from build123d import *

# Parameters (mm, degrees)
BOSS_EXTRUDE1_DEPTH = 20
SKETCH5_R           = 5.25
CUT_EXTRUDE4_DEPTH  = 20
SKETCH6_W           = 13
SKETCH6_H           = 13
CUT_EXTRUDE5_DEPTH  = 15.5
SKETCH7_W           = 13
SKETCH7_H           = 13
CUT_EXTRUDE6_DEPTH  = 15.5
SKETCH8_W           = 300
SKETCH8_H           = 102
BOSS_EXTRUDE2_DEPTH = 20
CUT_EXTRUDE7_START  = -150
SKETCH9_W           = 47.842391085
SKETCH9_H           = 20
CUT_EXTRUDE7_DEPTH  = 150
CUT_EXTRUDE9_DEPTH  = 40
CUT_EXTRUDE10_DEPTH = 60
SKETCH17_W          = 60
SKETCH17_H          = 5
CUT_EXTRUDE12_DEPTH = 38
CUT_EXTRUDE13_DEPTH = 60
SKETCH10_W          = 252.157608915
SKETCH10_H          = 50
CUT_EXTRUDE8_DEPTH  = 310
BOSS_EXTRUDE3_DEPTH = 50
SKETCH21_W          = 252.157608915
SKETCH21_H          = 10
CUT_EXTRUDE14_DEPTH = 54
SKETCH23_W          = 60
SKETCH23_H          = 5
BOSS_EXTRUDE5_DEPTH = 20
CUT_EXTRUDE15_DEPTH = 20
SKETCH22_W          = 60
SKETCH22_H          = 5
BOSS_EXTRUDE4_DEPTH = 20


with BuildPart() as part:
    # Sketch1 → Boss-Extrude1 (new body)
    with BuildSketch(Plane.XY):
        Polygon((-107.821386225, 92.09039548), (-7.821386225, 92.09039548), (117.178613775, 92.09039548), (117.178613775, 44.09039548), (-7.821386225, 44.09039548), (-107.821386225, 44.09039548), (-182.821386225, 44.09039548), (-182.821386225, 92.09039548), align=None)
    extrude(amount=BOSS_EXTRUDE1_DEPTH)

    # Sketch5 → Cut-Extrude4 (cut)
    with BuildSketch(Plane(origin=(0, 92.09039548, 0), x_dir=(1, 0, 0), z_dir=(0, 1, 0))):
        with Locations(Location((-66.321386225, -10, 0), (0, 0, 180))):
            Circle(SKETCH5_R)
        with Locations(Location((-47.321386225, -10, 0), (0, 0, 180))):
            Circle(SKETCH5_R)
    extrude(amount=-CUT_EXTRUDE4_DEPTH, mode=Mode.SUBTRACT)

    # Sketch6 → Cut-Extrude5 (cut)
    with BuildSketch(Plane(origin=(0, 92.09039548, 0), x_dir=(1, 0, 0), z_dir=(0, 1, 0))):
        with Locations((-99.441386225, -10.25)):
            Rectangle(SKETCH6_W, SKETCH6_H)
    extrude(amount=-CUT_EXTRUDE5_DEPTH, mode=Mode.SUBTRACT)

    # Sketch7 → Cut-Extrude6 (cut)
    with BuildSketch(Plane(origin=(0, 92.09039548, 0), x_dir=(1, 0, 0), z_dir=(0, 1, 0))):
        with Locations((-14.16377731, -10.25)):
            Rectangle(SKETCH7_W, SKETCH7_H)
    extrude(amount=-CUT_EXTRUDE6_DEPTH, mode=Mode.SUBTRACT)

    # Sketch8 → Boss-Extrude2 (add)
    with BuildSketch(Plane.XY.offset(20)):
        with Locations((-32.821386225, -6.90960452)):
            Rectangle(SKETCH8_W, SKETCH8_H)
    extrude(amount=-BOSS_EXTRUDE2_DEPTH)

    # Sketch9 → Cut-Extrude7 (cut)
    with BuildSketch(Plane(origin=(0, 92.09039548, 0), x_dir=(1, 0, 0), z_dir=(0, 1, 0)).offset(CUT_EXTRUDE7_START)):
        with Locations((93.257418233, -10)):
            Rectangle(SKETCH9_W, SKETCH9_H)
    extrude(amount=CUT_EXTRUDE7_DEPTH, mode=Mode.SUBTRACT)

    # Sketch11 → Cut-Extrude9 (cut)
    with BuildSketch(Plane.XY.offset(20)):
        Polygon((-26.742581768, 62.09039548), (-26.742581768, 12.09039548), (-86.742581768, 12.09039548), (-86.742581768, 62.09039548), (-86.742581768, 64.09039548), (-26.742581768, 64.09039548), align=None)
    extrude(amount=-CUT_EXTRUDE9_DEPTH, mode=Mode.SUBTRACT)

    # Sketch14 → Cut-Extrude10 (cut)
    with BuildSketch(Plane(origin=(-86.742581768, 0, 0), x_dir=(0, 0, -1), z_dir=(1, 0, 0))):
        Polygon((0, 64.09039548), (-20, 67.09039548), (-20, 64.09039548), align=None)
    extrude(amount=CUT_EXTRUDE10_DEPTH, mode=Mode.SUBTRACT)

    # Sketch17 → Cut-Extrude12 (cut)
    with BuildSketch(Plane(origin=(0, 0, 0), x_dir=(-1, 0, 0), z_dir=(0, 0, -1))):
        with Locations((56.742581768, 89.59039548)):
            Rectangle(SKETCH17_W, SKETCH17_H)
    extrude(amount=-CUT_EXTRUDE12_DEPTH, mode=Mode.SUBTRACT)

    # Sketch19 → Cut-Extrude13 (cut)
    with BuildSketch(Plane.ZY.offset(26.742581768)):
        Polygon((0, 12.09039548), (2, 12.09039548), (8, -57.90960452), (0, -57.90960452), align=None)
    extrude(amount=CUT_EXTRUDE13_DEPTH, mode=Mode.SUBTRACT)

    # Sketch10 → Cut-Extrude8 (cut)
    with BuildSketch(Plane(origin=(0, 0, 0), x_dir=(-1, 0, 0), z_dir=(0, 0, -1))):
        with Locations((56.742581767, -32.90960452)):
            Rectangle(SKETCH10_W, SKETCH10_H)
    extrude(amount=-CUT_EXTRUDE8_DEPTH, mode=Mode.SUBTRACT)

    # Sketch20 → Boss-Extrude3 (add)
    with BuildSketch(Plane.XZ.offset(7.90960452)):
        Polygon((69.33622269, 20), (-182.821386225, 20), (-182.821386225, 0), (-86.742581768, 0), (-86.742581768, 3.714285714), (-26.742581768, 3.714285714), (-26.742581768, 0), (69.33622269, 0), align=None)
    extrude(amount=BOSS_EXTRUDE3_DEPTH)

    # Sketch21 → Cut-Extrude14 (cut)
    with BuildSketch(Plane.XY.offset(20)):
        with Locations((-56.742581767, -52.90960452)):
            Rectangle(SKETCH21_W, SKETCH21_H)
    extrude(amount=-CUT_EXTRUDE14_DEPTH, mode=Mode.SUBTRACT)

    # Sketch23 → Boss-Extrude5 (add)
    with BuildSketch(Plane.XY.offset(20)):
        with Locations((-56.742581768, 89.59039548)):
            Rectangle(SKETCH23_W, SKETCH23_H)
    extrude(amount=-BOSS_EXTRUDE5_DEPTH)

    # Sketch24 → Cut-Extrude15 (cut)
    with BuildSketch(Plane.XY.offset(20)):
        Polygon((-86.742581768, 67.09039548), (-86.742581768, 72.09039548), (-26.742581768, 72.09039548), (-26.742581768, 67.09039548), (-26.742581768, 61.01073747), (-86.742581768, 61.01073747), align=None)
    extrude(amount=-CUT_EXTRUDE15_DEPTH, mode=Mode.SUBTRACT)

    # Sketch22 → Boss-Extrude4 (add)
    with BuildSketch(Plane.XY.offset(20)):
        with Locations((-56.742581768, 89.59039548)):
            Rectangle(SKETCH22_W, SKETCH22_H)
    extrude(amount=-BOSS_EXTRUDE4_DEPTH)


solid = part.part
For this review, take the finished solid that the model builds, in its own axes (mm). A direction names the side the tool comes from. Round coordinates to 2 decimals unless told otherwise and drop trailing zeros. Order: outer loops, then holes, each group sorted by start corner. A loop starts at its lowest first (then second) coordinate and runs counter-clockwise, first axis right, second up. Notation, with made-up numbers: M 83,63.25 L 141,63.25 A27 cw 141,99.25 Z; hole C 36,-21.5 d5. An arc over 180 degrees is marked long. Write each question's results on one line, items separated by ' | '. Start each with the question number.
1. To check wall thickness, follow L1, parallel to X at y = 68, z = 6.5; L2, parallel to Y at x = -79.5, z = 4.5; L3, parallel to Y at x = -71, z = 12. State the ranges of each line that lie inside material, in increasing order. Write a range as [from, to].
2. Add section C-C (y = 66). State the section outline as (x, z) points, then the cut area to 3 significant figures.
3. Tool access review of faces 4 (the face through (-100, 84, 3.75)), 5 (the face through (-57, 72.09, 10)), 6 (the face through (-71.33, 79.7, 11.58)): name each direction out of +Z, -Z, +X, -X, +Y, -Y from which nothing blocks a thin tool from reaching the whole face with its end or side.
4. Draft analysis for pull direction Z (two halves, no side actions). For faces 1 (the face through (-56.323, 2.23, 2.845)), 2 (the face through (-26.743, 26, 10)), 3 (the face through (-66, 87.09, 10)), state which applies: pulls with the +Z half, pulls with the -Z half, needs draft (parallel to the pull), parting line crosses it, or undercut.
5. Add section A-A (x = -79.5). State the section outline as (y, z) points.
6. Add section D-D (y = -33). State the section outline as (x, z) points.
7. Add section B-B (z = 10). State the section outline as (x, y) points.
Output values:
1) L1: [-182.82, -86.74], [-26.74, 69.34] | L2: [-47.91, 12.09], [72.09, 92.09] | L3: [-47.91, 12.09], [87.09, 92.09]
2) outline: M -182.82,0 L -86.74,0 L -86.74,20 L -182.82,20 Z; M -26.74,0 L 69.34,0 L 69.34,20 L -26.74,20 Z | area: 3,840 mm^2
3) face 4: +Y | face 5: +Z, -Z | face 6: none
4) face 1: pulls with the -Z half | face 2: needs draft | face 3: undercut
5) outline: M -47.91,3.71 L -7.91,3.71 L 12.09,2 L 12.09,20 L -47.91,20 Z; M 72.09,0 L 92.09,0 L 92.09,20 L 72.09,20 Z
6) outline: M -182.82,0 L -86.74,0 L -86.74,3.71 L -26.74,3.71 L -26.74,0 L 69.34,0 L 69.34,20 L -182.82,20 Z
7) outline: M -182.82,-47.91 L 69.34,-47.91 L 69.34,92.09 L -7.66,92.09 L -7.66,76.59 L -20.66,76.59 L -20.66,92.09 L -92.94,92.09 L -92.94,76.59 L -105.94,76.59 L -105.94,92.09 L -182.82,92.09 Z; hole M -86.74,12.09 L -26.74,12.09 L -26.74,72.09 L -42.07,72.09 L -42.07,87.09 L -52.57,87.09 L -52.57,72.09 L -61.07,72.09 L -61.07,87.09 L -71.57,87.09 L -71.57,72.09 L -86.74,72.09 Z
